Geometry: final body of the model. Coordinates: model frame, mm. A direction names the side the tool comes from. Coordinates: 2 decimals unless noted, no trailing zeros. Write each loop counter-clockwise with the first axis right and the second up, starting at its lowest first coordinate (ties: lowest second). Pieces come first, ordered by that corner, then holes. Notation, with made-up numbers: (-22, -3) -> (14, -3) arc R8 ccw to (14, 8) -> close; hole circle Ø9 at (4.25, -14). An arc over 180 degrees is marked (long way). Answer as a JSON object with one key per item and string values. Group by question number.
```python
from build123d import *

# Parameters (mm, degrees)
EXTRUDE_1_DEPTH     = 300
SHELL_2_T           = -5
CUT_EXTRUDE_1_DEPTH = 300
SKETCH_4_W          = 187.367155343
SKETCH_4_H          = 275.26588877
CUT_EXTRUDE_2_DEPTH = 10


with BuildPart() as part:
    # 草图1 → 凸台-拉伸1 (new body)
    with BuildSketch(Plane.XY):
        with BuildLine():
            Line((-402.186878728, -155.168986083), (297.813121272, -155.168986083))
            Line((297.813121272, -155.168986083), (297.813121272, -142.016461596))
            ThreePointArc((297.813121272, -142.016461596), (272.093642568, -75.065702407), (208.165038153, -42.553715721))
            Line((208.165038153, -42.553715721), (162.925157805, -37.845224347))
            Line((162.925157805, -37.845224347), (-44.606277086, 18.180372145))
            Line((-44.606277086, 18.180372145), (-120.025544077, 12.932974824))
            Line((-120.025544077, 12.932974824), (-370.712436241, -93.826427202))
            Line((-370.712436241, -93.826427202), (-383.529193777, -107.067800556))
            Line((-383.529193777, -107.067800556), (-402.186878728, -155.168986083))
        make_face()
    extrude(amount=EXTRUDE_1_DEPTH)

    # 抽壳2
    shell_2_openings = [part.faces().sort_by_distance(p)[0] for p in [
        (-52.186878728, -155.168986083, 150),
    ]]
    offset(amount=SHELL_2_T, openings=shell_2_openings, kind=Kind.INTERSECTION)

    # 草图3 → 切除-拉伸1 (cut)
    with BuildSketch(Plane(origin=(0, 0, 0), x_dir=(-1, 0, 0), z_dir=(0, 0, -1))):
        Polygon((145.146298651, -44.9212837), (128.165102127, 0), (335.819907539, -89.355551576), (185.513355718, -73.15629574), align=None)
        Polygon((107.735938101, 3.900733264), (125.333088077, -44.9212837), (104.080540111, -73.15629574), (-59.15944036, -73.15629574), (-148.825386801, -43.221714567), (46.237805698, 9.665692949), align=None)
    extrude(amount=-CUT_EXTRUDE_1_DEPTH, mode=Mode.SUBTRACT)

    # 草图4 → 切除-拉伸2 (cut)
    with BuildSketch(Plane(origin=(1.544560656, 5.721400739, 0), x_dir=(0.9654383198530997, -0.26063163767897407, 0), z_dir=(0.26063163767897407, 0.9654383198530997, 0))):
        with Locations((61.249747997, -149.050418092)):
            Rectangle(SKETCH_4_W, SKETCH_4_H)
    extrude(amount=-CUT_EXTRUDE_2_DEPTH, mode=Mode.SUBTRACT)


solid = part.part
```
Item 1: Section B-B on x = 42. Output: boundary loops of the cut face in (y, z), then the cut area to 3 significant figures.
Item 2: Set-up query: faces 5 (the flat face through (297.813, -149, 148)), 6 (the flat face through (-114.856, -58.841, 2.465)), 7 (the flat face through (-57, -107, 295)). Return all of +Z, -Z, +X, -X, +Y, -Y with unobstructed straight access to the full face (end or side cutting, diameter ignored); none if empty.
Item 3: Section C-C on x = -237.5. Output: boundary loops of the cut face in (y, z), then the cut area to 3 significant figures.
Item 4: Contact query for flat-ended pins moving along their axis: pin 1 (3 mm diameter, centred on y = -132, z = 145, fed in from -X); pin 2 (2.5 mm diameter, centred on x = -41, z = 298, fed in from +Y); pin 3 (4 mm diameter, centred on y = -123.5, z = 84.5, fed in from -X). Output: stop coordinate, or through.
Item 5: Section A-A on z = 269. Output: boundary loops of the cut face in (x, y).
Item 6: Mould query, pull axis Z, two halves, no side actions, for faces 1 (the cylindrical face through (269.03, -79.14, 147.97)), 2 (the flat face through (-243.614, -39.699, 147.9)), 3 (the flat face through (-57, -106, 0)), 4 (the flat face through (-57, -106, 300)). Classes: +Z half, -Z half, draft (parallel to the pull), parting line (faces both ways), or undercut.
Item 7: Section D-D on y = -21. Output: boundary loops of the cut face in (x, z).
Item 8: Ray query, L1, parallel to Z at x = 169.5, y = -131; L2, parallel to X at y = -106.5, z = 96; L3, parallel to X at y = -86, z = 28. Return the intervals inside material, ascending. Write a range as [from, to].
Answer sheet:
{
 "1": {"outline": "(-155.17, 0) -> (-73.16, 0) -> (-73.16, 5) -> (-155.17, 5) -> close; (-155.17, 295) -> (-73.16, 295) -> (-73.16, 300) -> (-155.17, 300) -> close; (-14.26, 0) -> (-5.2, 0) -> (-5.2, 11.42) -> (-10.38, 11.42) -> (-10.38, 5) -> (-14.26, 5) -> close; (-14.26, 295) -> (-10.38, 295) -> (-10.38, 286.68) -> (-5.2, 286.68) -> (-5.2, 300) -> (-14.26, 300) -> close", "area": "987 mm^2"},
 "2": {"face 5": "+Z, -Z, +X, +Y, -Y", "face 6": "+Z, -Z", "face 7": "-Y"},
 "3": {"outline": "(-155.17, 0) -> (-78.76, 0) -> (-78.76, 5) -> (-155.17, 5) -> close; (-155.17, 295) -> (-78.76, 295) -> (-78.76, 300) -> (-155.17, 300) -> close; (-47.05, 0) -> (-37.1, 0) -> (-37.1, 300) -> (-47.05, 300) -> (-47.05, 295) -> (-42.53, 295) -> (-42.53, 5) -> (-47.05, 5) -> close", "area": "2,440 mm^2"},
 "4": {"pin 1": "stops at x = -393.78", "pin 2": "stops at y = 17.54", "pin 3": "stops at x = -390.68"},
 "5": {"outline": "(-402.19, -155.17) -> (-396.82, -155.17) -> (-379.23, -109.82) -> (-367.82, -98.03) -> (-118.84, 8) -> (-45.1, 13.13) -> (-31.07, 9.35) -> (-29.77, 14.17) -> (-44.61, 18.18) -> (-120.03, 12.93) -> (-370.71, -93.83) -> (-383.53, -107.07) -> close; (149.82, -39.49) -> (162.01, -42.78) -> (207.65, -47.53) arc R95 cw to (292.81, -142.02) -> (292.81, -155.17) -> (297.81, -155.17) -> (297.81, -142.02) arc R100 ccw to (208.17, -42.55) -> (162.93, -37.85) -> (151.12, -34.66) -> close"},
 "6": {"face 1": "undercut", "face 2": "draft", "face 3": "-Z half", "face 4": "+Z half"},
 "7": {"outline": "(-199.71, 0) -> (-176.97, 0) -> (-176.97, 5) -> (-186.94, 5) -> (-186.94, 295) -> (-176.97, 295) -> (-176.97, 300) -> (-199.71, 300) -> close; (-136.1, 0) -> (-116.71, 0) -> (-116.71, 5) -> (-136.1, 5) -> close; (-136.1, 295) -> (-116.71, 295) -> (-116.71, 300) -> (-136.1, 300) -> close; (66.87, 0) -> (100.53, 0) -> (100.53, 11.42) -> (81.34, 11.42) -> (81.34, 5) -> (66.87, 5) -> close; (66.87, 295) -> (81.34, 295) -> (81.34, 286.68) -> (100.53, 286.68) -> (100.53, 300) -> (66.87, 300) -> close"},
 "8": {"L1": "z = [0, 5], [295, 300]", "L2": "x = [-382.98, -376.02], [285.92, 291.29]", "L3": "x = [-352.33, -339.57], [274.54, 280.65]"}
}
